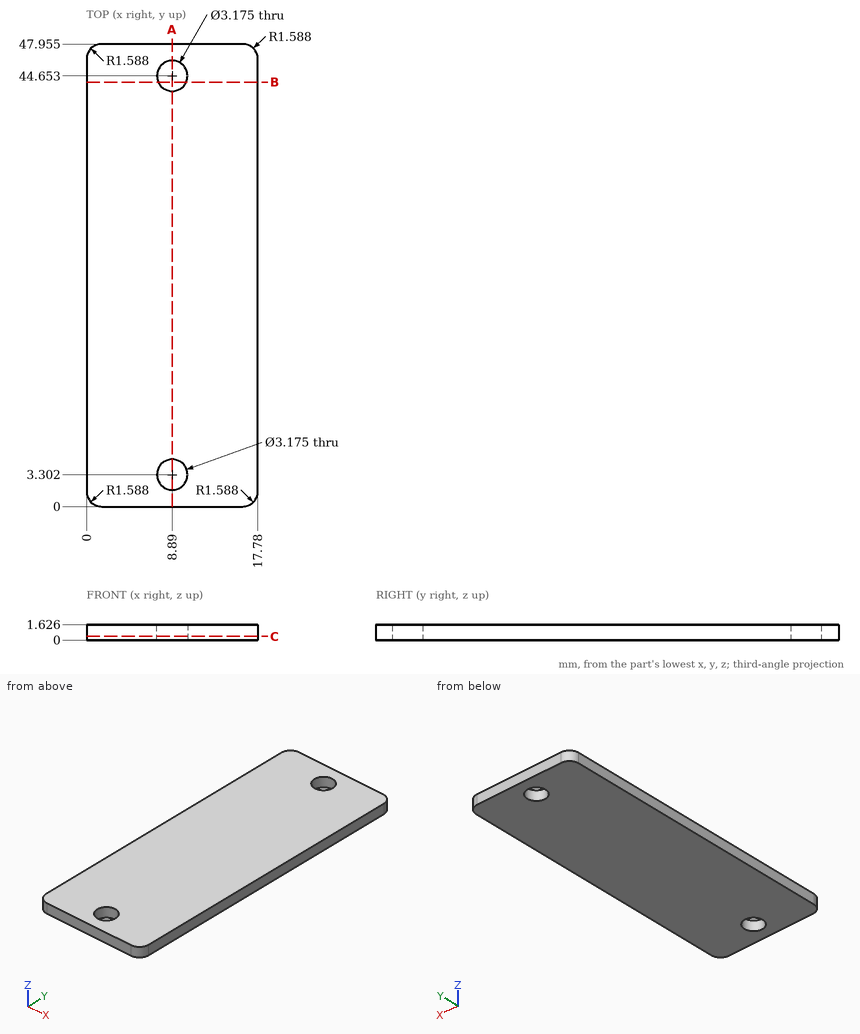
Design review of the part shown in the three views and the two pictorial views. Dimensions are in mm from the part's minimum x, y and z. Coordinates: 2 decimals unless noted, no trailing zeros. Loops run counter-clockwise (first coordinate to the right, second up) from the corner with the lowest first, then second, coordinate; pieces in that order, holes last.
(1) Wall thickness on L1, parallel to Y at x = 8.89, z = 0.4 (1 decimal); L2, parallel to Y at x = 9.75, z = 1 (1 decimal); L3, parallel to X at y = 46, z = 0.75: over which ranges is each line inside the solid? List them lowest first.
Determined:
L1: y = 0 to 1.7, 4.9 to 43.1, 46.2 to 48
L2: y = 0 to 2, 4.6 to 43.3, 46 to 48
L3: x = 0 to 8.05, 9.73 to 17.78
(2) Consider section A-A, the plane x = 8.89. Give the boundary of the cut face in (y, z) (1 decimal).
Determined:
outline: (0, 0) - (1.7, 0) - (1.7, 1.6) - (0, 1.6) - close; (4.9, 0) - (43.1, 0) - (43.1, 1.6) - (4.9, 1.6) - close; (46.2, 0) - (48, 0) - (48, 1.6) - (46.2, 1.6) - close
(3) Insertion check: P1, Ø3, axis at x = 5.5, y = 40.5, coming from the -Z side. The pin has a flat end and moves straight along its axis. Give the tip position at first contact, or say it passes through.
Determined:
P1: stops at z = 0
(4) Consider section C-C, the plane z = 0.4. Give the boundary of the cut face in (x, y) (1 decimal).
Determined:
outline: (0, 1.6) arc R1.6 ccw to (1.6, 0) - (16.2, 0) arc R1.6 ccw to (17.8, 1.6) - (17.8, 46.4) arc R1.6 ccw to (16.2, 48) - (1.6, 48) arc R1.6 ccw to (0, 46.4) - close; hole circle Ø3.2 at (8.9, 3.3); hole circle Ø3.2 at (8.9, 44.7)
(5) Consider section B-B, the plane y = 44. Give the boundary of the cut face in (x, z) (1 decimal), plus the area to 3 significant figures.
Determined:
outline: (0, 0) - (7.4, 0) - (7.4, 1.6) - (0, 1.6) - close; (10.3, 0) - (17.8, 0) - (17.8, 1.6) - (10.3, 1.6) - close
area: 24.2 mm2
